Geometry: final body of the model. Coordinates: model frame, mm. Give positions to 0.01 mm unless a question says otherwise; leave off trailing zeros. Write each loop counter-clockwise with the first axis right and the second up, starting at its lowest first coordinate (ties: lowest second). Pieces come first, ordered by that corner, then holes.
from build123d import *

# Parameters (mm, degrees)
SKETCH1_W           = 132.132132132
SKETCH1_H           = 100
BOSS_EXTRUDE1_DEPTH = 15
SKETCH2_R           = 4
CUT_EXTRUDE1_DEPTH  = 20
FILLET1_R           = 3


with BuildPart() as part:
    # Sketch1 → Boss-Extrude1 (new body)
    with BuildSketch(Plane.XY):
        Rectangle(SKETCH1_W, SKETCH1_H)
    extrude(amount=BOSS_EXTRUDE1_DEPTH)

    # Sketch2 → Cut-Extrude1 (cut)
    with BuildSketch(Plane.XZ.offset(50)):
        with Locations(Location((-54.066066066, 7.5, 0), (0, 0, 270))):
            Circle(SKETCH2_R)
        with Locations(Location((54.066066066, 7.5, 0), (0, 0, 90))):
            Circle(SKETCH2_R)
    cut_extrude1 = extrude(amount=-CUT_EXTRUDE1_DEPTH, mode=Mode.SUBTRACT)

    # Mirror1: Cut-Extrude1 across plane
    add(cut_extrude1.mirror(Plane.ZX), mode=Mode.SUBTRACT)

    # Fillet1
    fillet1_edges = [part.edges().sort_by_distance(p)[0] for p in [
        (-66.066066066, 0, 15),
        (0, -50, 15),
        (66.066066066, 0, 15),
        (0, -50, 0),
        (-66.066066066, 0, 0),
        (0, 50, 0),
        (66.066066066, 0, 0),
        (66.066066066, -50, 7.5),
        (-66.066066066, -50, 7.5),
        (-66.066066066, 50, 7.5),
        (66.066066066, 50, 7.5),
        (0, 50, 15),
    ]]
    fillet(fillet1_edges, radius=FILLET1_R)


solid = part.part
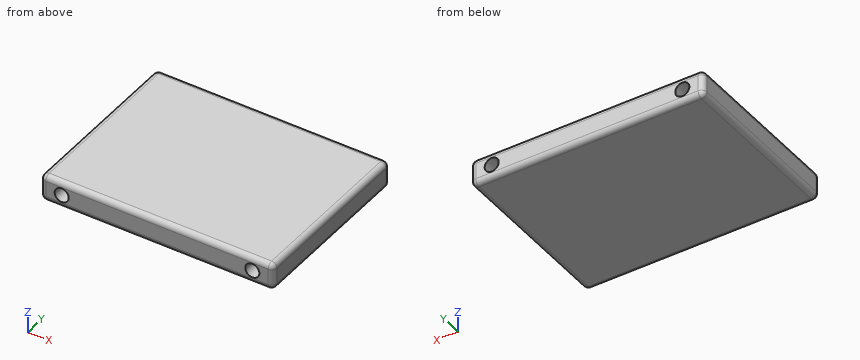
Q1. Pin query (flat end, axial travel): P1, Ø6.5, axis at x = -56, z = 8, coming from the +Y side; P2, Ø2.5, axis at x = 53.5, z = 6.5, coming from the -Y side; P3, Ø4, axis at x = 54, z = 6, coming from the +Y side. Return the tip coordinate at first contact, or that it passes through.
Filled sheet:
P1: stops at y = 50
P2: stops at y = -30
P3: stops at y = 30
Q2. Ray query, line 1 along X through (y, z) = (34.75, 7.5); line 2 along X through (y, z) = (-41.5, 10.75); line 3 along Y through (x, z) = (-25, 2.75). Return the intervals inside material, ascending.
Filled sheet:
line 1: x = -66.07 to -58.07, -50.07 to 50.07, 58.07 to 66.07
line 2: x = -66.07 to -56.4, -51.73 to 51.73, 56.4 to 66.07
line 3: y = -49.99 to 49.99
Q3. Section A-A on z = 7.5. Output: boundary loops of the cut face in (x, y).
Filled sheet:
outline: (-66.07, -47) arc R3 ccw to (-63.07, -50) - (-58.07, -50) - (-58.07, -30) - (-50.07, -30) - (-50.07, -50) - (50.07, -50) - (50.07, -30) - (58.07, -30) - (58.07, -50) - (63.07, -50) arc R3 ccw to (66.07, -47) - (66.07, 47) arc R3 ccw to (63.07, 50) - (58.07, 50) - (58.07, 30) - (50.07, 30) - (50.07, 50) - (-50.07, 50) - (-50.07, 30) - (-58.07, 30) - (-58.07, 50) - (-63.07, 50) arc R3 ccw to (-66.07, 47) - close
Q4. Section B-B on y = -41. Output: boundary loops of the cut face in (x, z).
Filled sheet:
outline: (-66.07, 3) arc R3 ccw to (-63.07, 0) - (63.07, 0) arc R3 ccw to (66.07, 3) - (66.07, 12) arc R3 ccw to (63.07, 15) - (-63.07, 15) arc R3 ccw to (-66.07, 12) - close; hole circle Ø8 at (-54.07, 7.5); hole circle Ø8 at (54.07, 7.5)
